Check sheet for the drawn part. Datum: minimum x, y, z corner. Units: mm. A direction names the side the tool comes from. Round coordinates to 2 decimals unless told otherwise and drop trailing zeros. Write each loop counter-clockwise with the first axis right and the second up, starting at its lowest first coordinate (ties: lowest second). Pieces come first, ordered by that corner, then holes.
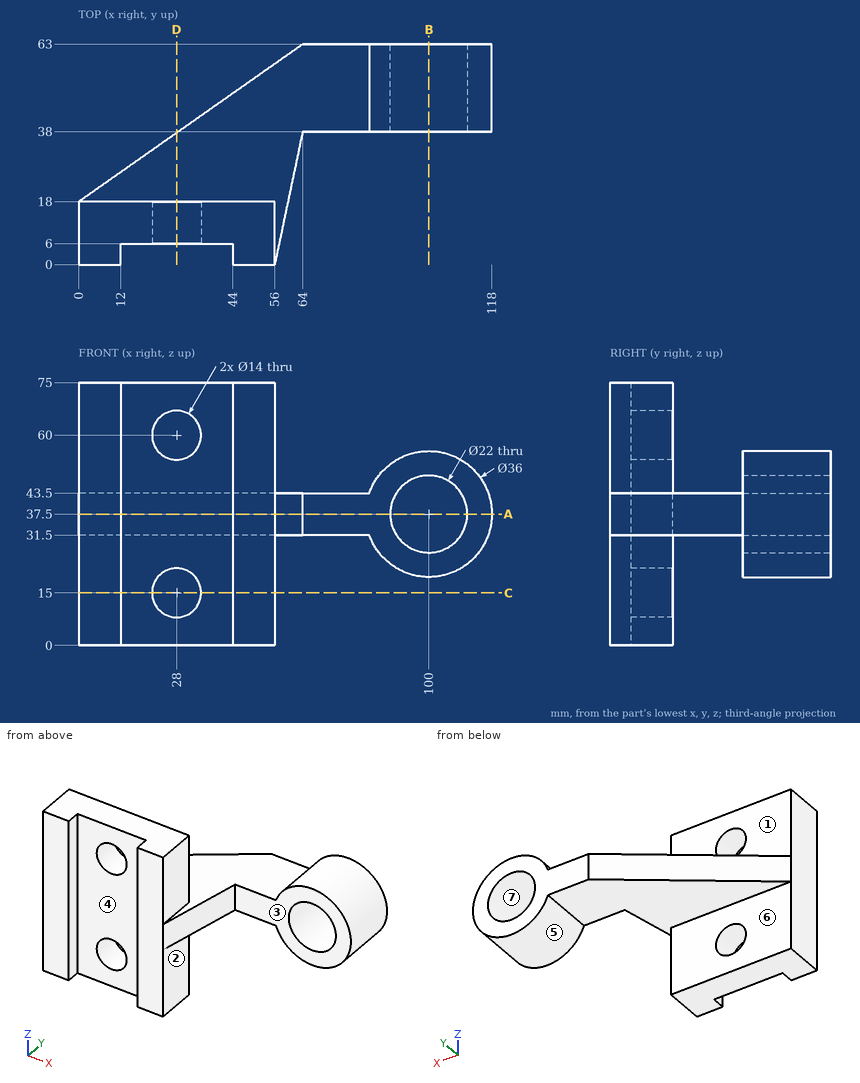
Q1. Sectioned sample at B-B (x = 100). Enter the section's corners in (y, z).
Recorded:
outline: (38, 19.5) - (63, 19.5) - (63, 26.5) - (38, 26.5) - close; (38, 48.5) - (63, 48.5) - (63, 55.5) - (38, 55.5) - close
Q2. Sectioned sample at D-D (x = 28). Enter the section's corners in (y, z), plus the area to 3 significant figures.
Recorded:
outline: (6, 0) - (18, 0) - (18, 8) - (6, 8) - close; (6, 22) - (18, 22) - (18, 31.5) - (37.69, 31.5) - (37.69, 43.5) - (18, 43.5) - (18, 53) - (6, 53) - close; (6, 67) - (18, 67) - (18, 75) - (6, 75) - close
area: 800 mm2
Q3. Tool access check on the marked faces 1, 2, 3 and 4. Record the directions out of +Z, -Z, +X, -X, +Y, -Y that give a thin tool (end or side, any length) a straight path to the whole face; none if there is none.
Recorded:
face 1: +Z, +X, -X, +Y
face 2: -Z, +X, +Y, -Y
face 3: +Z, -Z, +X, -Y
face 4: +Z, -Z, -Y
Q4. Sectioned sample at A-A (z = 37.5). Enter the section's corners in (x, y).
Recorded:
outline: (0, 0) - (12, 0) - (12, 6) - (44, 6) - (44, 0) - (56, 0) - (64, 38) - (89, 38) - (89, 63) - (64, 63) - (0, 18) - close; (111, 38) - (118, 38) - (118, 63) - (111, 63) - close
Q5. Release check for a two-part mould opening along X. For the marked faces 5, 6 and 7 record: released by +X, released by -X, zero draft, split by the parting line, or undercut.
Recorded:
face 5: split by the parting line
face 6: zero draft
face 7: undercut
Q6. Material ranges on line 1 along Z through (x, y) = (28, 13); line 2 along X through (y, z) = (4, 3); line 3 along X through (y, z) = (13.25, 60), recorded low to high.
Recorded:
line 1: z = 0 to 8, 22 to 53, 67 to 75
line 2: x = 0 to 12, 44 to 56
line 3: x = 0 to 21, 35 to 56
Q7. Depth check by flat-ended pin: P1, Ø8, axis at x = 23, z = 35, coming from the +Y side; P2, Ø2, axis at x = 15, z = 59, coming from the +Y side; P3, Ø9.5, axis at x = 27, z = 44.5, coming from the -Y side. Enter the tip coordinate at first touch or a pass-through.
Recorded:
P1: stops at y = 36.98
P2: stops at y = 18
P3: stops at y = 6
Q8. Sectioned sample at C-C (z = 15). Enter the section's corners in (x, y), plus the area to 3 significant figures.
Recorded:
outline: (0, 0) - (12, 0) - (12, 6) - (21, 6) - (21, 18) - (0, 18) - close; (35, 6) - (44, 6) - (44, 0) - (56, 0) - (56, 18) - (35, 18) - close
area: 648 mm2
